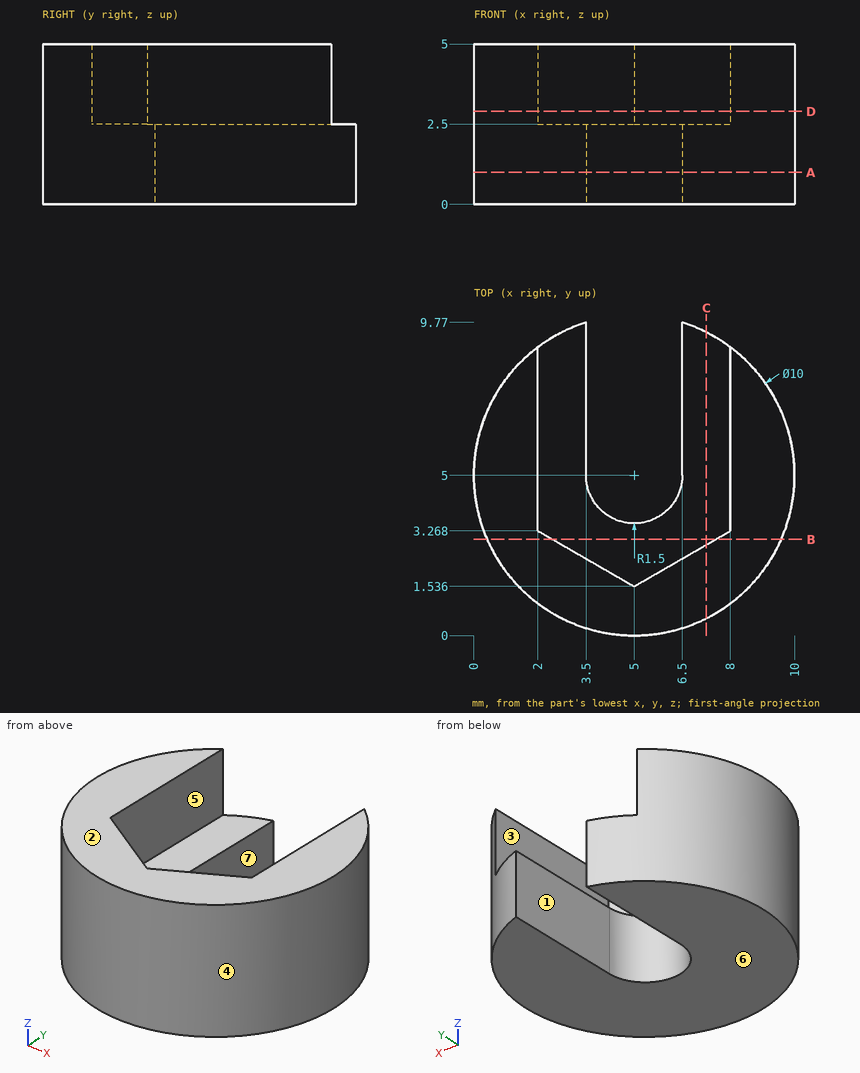
For this review, use the dimensioned drawing (mm, ordinates from the lowest corner) and the shaded views. A direction names the side the tool comes from. Round coordinates to 2 decimals unless told otherwise and drop trailing zeros. Write each loop counter-clockwise with the first axis right and the second up, starting at its lowest first coordinate (ties: lowest second). Pieces come first, ordered by that corner, then holes. Notation, with made-up numbers: (-27, 54.25) -> (-5, 54.25) arc R16 cw to (-5, 75.25) -> close; hole circle Ø1 at (70.5, -18.5). An arc over 180 degrees is marked (long way). One line per item, written item: value. Start each with the question number.
Q1. Add section A-A (z = 1). Give the boundary of the cut face in (x, y).
Q2. Add section C-C (x = 7.25). Give the boundary of the cut face in (y, z) (1 decimal), then the cut area to 3 significant figures.
Q3. The part is to be moulded in two halves that separate along X. For the marked faces 1, 2, 3 and 4, say which applies: pulls with the +X half, pulls with the -X half, needs draft (parallel to the pull), parting line crosses it, or undercut.
Q4. Add section D-D (z = 2.9). Give the boundary of the cut face in (x, y).
Q5. Tool access review of the marked faces 5, 6 and 7: name each direction out of +Z, -Z, +X, -X, +Y, -Y from which nothing blocks a thin tool from reaching the whole face with its end or side.
Q6. Insertion check: P1, Ø2, axis at y = 6.5, z = 1, coming from the +X side (3 decimals); P2, Ø1.2, axis at y = 7.5, z = 4, coming from the +X side (1 decimal); P3, Ø0.8, axis at y = 6.5, z = 4, coming from the -X side. Each pin has a flat end and moves straight along its axis. Give the tip position at first contact, or say it passes through.
Q7. To check wall thickness, follow probe 1 along Z at (x, y) = (7.25, 8.5); probe 2 along X at (y, z) = (4.75, 4.55); probe 3 along X at (y, z) = (1, 0.35). State the ranges of each line that lie inside material, in increasing order.
Q8. Add section B-B (y = 3). Give the boundary of the cut face in (x, z).
Response:
1. outline: (3.5, 5) -> (3.5, 9.77) arc R5 ccw (long way) to (6.5, 9.77) -> (6.5, 5) arc R1.5 cw to start
2. outline: (0.5, 0) -> (9.5, 0) -> (9.5, 2.5) -> (2.8, 2.5) -> (2.8, 5) -> (0.5, 5) -> close
2. area: 28.1 mm^2
3. face 1: undercut
3. face 2: needs draft
3. face 3: undercut
3. face 4: parting line crosses it
4. outline: (2, 3.27) -> (2, 9) arc R5 ccw (long way) to (8, 9) -> (8, 3.27) -> (5, 1.54) -> close
5. face 5: +Z, +Y
5. face 6: -Z, +X, -X, +Y, -Y
5. face 7: +Z, -Z, +Y
6. P1: stops at x = 9.975
6. P2: stops at x = 9.6
6. P3: stops at x = 0.12
7. probe 1: z = 0 to 2.5
7. probe 2: x = 0.01 to 2, 8 to 9.99
7. probe 3: x = 2 to 8
8. outline: (0.42, 0) -> (9.58, 0) -> (9.58, 5) -> (7.54, 5) -> (7.54, 2.5) -> (2.46, 2.5) -> (2.46, 5) -> (0.42, 5) -> close
